Design review of the part built by this model. Coordinates are the model's own, in mm. A direction names the side the tool comes from. Give positions to 0.01 mm unless a question says otherwise; leave off trailing zeros. Order: outer loops, then holes, each group sorted by start corner. A loop starts at its lowest first (then second) coordinate and runs counter-clockwise, first axis right, second up.
```python
from build123d import *

# Parameters (mm, degrees)
F0_W      = 115
F0_H      = 40
F1_DEPTH  = 12
F3_DEPTH  = 12.1
F4_R      = 3.15
F5_DEPTH  = 12.1
F6_R      = 5.5
F7_DEPTH  = 7
F8_R      = 3.3
F9_DEPTH  = 40.1
F10_R     = 5.5
F11_DEPTH = 8


with BuildPart() as f1:
    # F0 (on Top) → F1 (new body)
    with BuildSketch(Plane.XY):
        with Locations((57.5, -20)):
            Rectangle(F0_W, F0_H)
    extrude(amount=F1_DEPTH)

    # F2 (on Top) → F3 (cut)
    with BuildSketch(Plane.XY):
        with BuildLine():
            Line((30.75, -24.5), (30.75, -14.5))
            ThreePointArc((30.75, -14.5), (27.5, -11.25), (24.25, -14.5))
            Line((24.25, -14.5), (24.25, -24.5))
            ThreePointArc((24.25, -24.5), (27.5, -27.75), (30.75, -24.5))
        make_face()
        with BuildLine():
            ThreePointArc((60.75, -14.5), (57.5, -11.25), (54.25, -14.5))
            Line((54.25, -14.5), (54.25, -24.5))
            ThreePointArc((54.25, -24.5), (57.5, -27.75), (60.75, -24.5))
            Line((60.75, -24.5), (60.75, -14.5))
        make_face()
        with BuildLine():
            ThreePointArc((90.75, -14.5), (87.5, -11.25), (84.25, -14.5))
            Line((84.25, -14.5), (84.25, -24.5))
            ThreePointArc((84.25, -24.5), (87.5, -27.75), (90.75, -24.5))
            Line((90.75, -24.5), (90.75, -14.5))
        make_face()
    extrude(amount=F3_DEPTH, mode=Mode.SUBTRACT)

    # F4 (on Top) → F5 (cut)
    with BuildSketch(Plane.XY):
        with Locations((6, -7)):
            Circle(F4_R)
        with Locations((6, -33)):
            Circle(F4_R)
        with BuildLine():
            ThreePointArc((109, -10.15), (111.227386, -9.227386), (112.15, -7))
            ThreePointArc((112.15, -7), (106.772614, -4.772614), (109, -10.15))
        make_face()
        with BuildLine():
            ThreePointArc((112.15, -33), (111.227386, -30.772614), (109, -29.85))
            ThreePointArc((109, -29.85), (106.772614, -35.227386), (112.15, -33))
        make_face()
    extrude(amount=F5_DEPTH, mode=Mode.SUBTRACT)

    # F6 (on face) → F7 (cut)
    with BuildSketch(Plane.XY.offset(12)):
        with Locations((6, -7)):
            Circle(F6_R)
        with Locations((6, -33)):
            Circle(F6_R)
        with Locations((109, -7)):
            Circle(F6_R)
        with Locations((109, -33)):
            Circle(F6_R)
    extrude(amount=-F7_DEPTH, mode=Mode.SUBTRACT)

    # F8 (on face) → F9 (cut)
    with BuildSketch(Plane.XZ.offset(40)):
        with Locations((97, 6)):
            Circle(F8_R)
        with Locations((18, 6)):
            Circle(F8_R)
    extrude(amount=-F9_DEPTH, mode=Mode.SUBTRACT)

    # F10 (on face) → F11 (cut)
    with BuildSketch(Plane.XZ.offset(40)):
        with Locations((18, 6)):
            Circle(F10_R)
        with Locations((97, 6)):
            Circle(F10_R)
    extrude(amount=-F11_DEPTH, mode=Mode.SUBTRACT)


solid = f1.part
```
1. For line 1 along Y through (x, z) = (109, 3.4); line 2 along X through (y, z) = (-14.5, 11.5); line 3 along X through (y, z) = (-6, 2.25), list the stretches that pass through material, from the lowest coordinate up.
Recorded:
line 1: y = -40 to -36.15, -29.85 to -10.15, -3.85 to 0
line 2: x = 0 to 24.25, 30.75 to 54.25, 60.75 to 84.25, 90.75 to 115
line 3: x = 0 to 3.01, 8.99 to 106.01, 111.99 to 115
2. For pin 1 (3.5 mm diameter, centred on x = 107.5, y = -32, fed in from +Z), flat-tipped, find the tip position at first contact; note if it passes through.
Recorded:
pin 1: stops at z = 5
3. Take a section at B-B (x = 6). State the section outline as (y, z) points.
Recorded:
outline: (-40, 0) - (-36.15, 0) - (-36.15, 5) - (-38.5, 5) - (-38.5, 12) - (-40, 12) - close; (-29.85, 0) - (-10.15, 0) - (-10.15, 5) - (-12.5, 5) - (-12.5, 12) - (-27.5, 12) - (-27.5, 5) - (-29.85, 5) - close; (-3.85, 0) - (0, 0) - (0, 12) - (-1.5, 12) - (-1.5, 5) - (-3.85, 5) - close
4. Machinability: for faces 5 (the face through (16.81, -36.06, 0.63)), 6 (the face through (5.284, -27.547, 8.549)), 7 (the face through (30.75, -20, 6)), 8 (the face through (93.7, -16.2, 6.1)), which of the approach directions +Z, -Z, +X, -X, +Y, -Y give a long, thin tool a straight path to every point of the face, cutting with its end or side? Answer none if there is none.
Recorded:
face 5: -Y
face 6: +Z
face 7: +Z, -Z
face 8: +Y, -Y
5. Take a section at A-A (y = -16.5). State the section outline as (x, z) points.
Recorded:
outline: (0, 0) - (24.25, 0) - (24.25, 12) - (0, 12) - close; (30.75, 0) - (54.25, 0) - (54.25, 12) - (30.75, 12) - close; (60.75, 0) - (84.25, 0) - (84.25, 12) - (60.75, 12) - close; (90.75, 0) - (115, 0) - (115, 12) - (90.75, 12) - close; hole circle Ø6.6 at (18, 6); hole circle Ø6.6 at (97, 6)
6. Take a section at D-D (z = 10.5). State the section outline as (x, y) points.
Recorded:
outline: (0, -40) - (14.84, -40) - (14.84, -32) - (21.16, -32) - (21.16, -40) - (93.84, -40) - (93.84, -32) - (100.16, -32) - (100.16, -40) - (115, -40) - (115, 0) - (0, 0) - close; hole circle Ø11 at (6, -33); hole circle Ø11 at (6, -7); hole (24.25, -24.5) arc R3.25 ccw to (30.75, -24.5) - (30.75, -14.5) arc R3.25 ccw to (24.25, -14.5) - close; hole (54.25, -24.5) arc R3.25 ccw to (60.75, -24.5) - (60.75, -14.5) arc R3.25 ccw to (54.25, -14.5) - close; hole (84.25, -24.5) arc R3.25 ccw to (90.75, -24.5) - (90.75, -14.5) arc R3.25 ccw to (84.25, -14.5) - close; hole circle Ø11 at (109, -33); hole circle Ø11 at (109, -7)
7. Take a section at C-C (x = 27.5). State the section outline as (y, z) points.
Recorded:
outline: (-40, 0) - (-27.75, 0) - (-27.75, 12) - (-40, 12) - close; (-11.25, 0) - (0, 0) - (0, 12) - (-11.25, 12) - close
8. Draft analysis for pull direction X (two halves, no side actions). For faces 1 (the face through (115, -20, 6)), 2 (the face through (0, -20, 6)), 3 (the face through (57, -11, 12)), 4 (the face through (7.69, -4.34, 2.46)), state which applies: pulls with the +X half, pulls with the -X half, needs draft (parallel to the pull), parting line crosses it, or undercut.
Recorded:
face 1: pulls with the +X half
face 2: pulls with the -X half
face 3: needs draft
face 4: undercut
